from build123d import *

# Parameters (mm, degrees)
SKIZZE1_W                                 = 25
SKIZZE1_H                                 = 24
PCB_DEPTH                                 = 0.9
SKIZZE2_R                                 = 1.05
MOUNTING_HOLES_DEPTH                      = 20.165333287
SKIZZE3_W                                 = 20.8
SKIZZE3_H                                 = 5.5
CONNECTOR_CLOSED_DEPTH                    = 2.4
SKIZZE4_W                                 = 17.7
SKIZZE4_H                                 = 11.6
COMPONENTS_WORST_CASE_BOUNDARY_BOX_DEPTH  = 1.3
SKIZZE7_W                                 = 3
SKIZZE7_H                                 = 2
COMPONENTS_WORST_CASE_BOUNDARY_BOX2_DEPTH = 0.6
SKIZZE8_W                                 = 1.3
SKIZZE8_H                                 = 0.9
STATUS_LED_DEPTH                          = 0.01
ESBO_O1_R                                 = 3.5
RESSALTO_EXTRUS_O2_DEPTH                  = 3


with BuildPart() as part:
    # Skizze1 → PCB (new body)
    with BuildSketch(Plane(origin=(0, 0, 0), x_dir=(1, 0, 0), z_dir=(0, 1, 0))):
        with Locations((0, 2.5)):
            Rectangle(SKIZZE1_W, SKIZZE1_H)
    extrude(amount=-PCB_DEPTH)

    # Skizze2 → Mounting_Holes (cut, through all)
    with BuildSketch(Plane(origin=(0, 0, 0), x_dir=(1, 0, 0), z_dir=(0, 1, 0))):
        with Locations(Location((10.5, 12.5, 0), (0, 0, 270))):
            Circle(SKIZZE2_R)
        with Locations(Location((10.5, 0, 0), (0, 0, 270))):
            Circle(SKIZZE2_R)
        with Locations(Location((-10.5, 0, 0), (0, 0, 90))):
            Circle(SKIZZE2_R)
        with Locations(Location((-10.5, 12.5, 0), (0, 0, 90))):
            Circle(SKIZZE2_R)
    extrude(amount=-MOUNTING_HOLES_DEPTH, mode=Mode.SUBTRACT)

    # Skizze3 → Connector_closed (add)
    with BuildSketch(Plane.XZ.offset(0.9)):
        with Locations((0, 6.75)):
            Rectangle(SKIZZE3_W, SKIZZE3_H)
    extrude(amount=CONNECTOR_CLOSED_DEPTH)

    # Skizze4 → Components_worst-case_Boundary-Box (add)
    with BuildSketch(Plane.XZ.offset(0.9)):
        with Locations((-0.15, -6.7)):
            Rectangle(SKIZZE4_W, SKIZZE4_H)
    extrude(amount=COMPONENTS_WORST_CASE_BOUNDARY_BOX_DEPTH)

    # Skizze7 → Components_worst-case_Boundary-Box2 (add)
    with BuildSketch(Plane(origin=(0, 0, 0), x_dir=(1, 0, 0), z_dir=(0, 1, 0))):
        with Locations((7, 9.9)):
            Rectangle(SKIZZE7_W, SKIZZE7_H)
    extrude(amount=COMPONENTS_WORST_CASE_BOUNDARY_BOX2_DEPTH)

    # Skizze8 → Status_LED (cut)
    with BuildSketch(Plane(origin=(0, 0.6, 0), x_dir=(1, 0, 0), z_dir=(0, 1, 0))):
        with Locations((7.45, 9.45)):
            Rectangle(SKIZZE8_W, SKIZZE8_H)
    extrude(amount=-STATUS_LED_DEPTH, mode=Mode.SUBTRACT)

    # Esboço1 → Ressalto-extrusão2 (add)
    with BuildSketch(Plane(origin=(0, 0, 0), x_dir=(1, 0, 0), z_dir=(0, 1, 0))):
        with Locations(Location((0, 0, 0), (0, 0, 270))):
            Circle(ESBO_O1_R)
    extrude(amount=RESSALTO_EXTRUS_O2_DEPTH)


solid = part.part
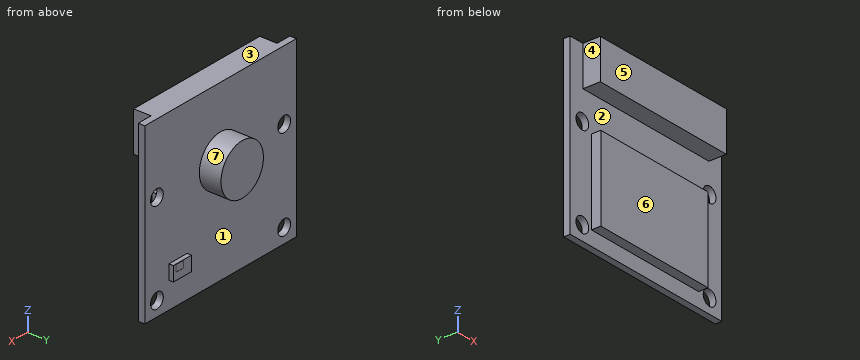
Could you check a few things on this model? Use its own coordinates, in mm. Face numbers are marked on the shaded views. A direction names the side the tool comes from. Coordinates: 2 decimals unless noted, no trailing zeros. Write each loop counter-clockwise with the first axis right and the second up, starting at its lowest first coordinate (ties: lowest second). Pieces come first, ordered by that corner, then holes. Notation, with made-up numbers: (61, 22) - (87, 22) arc R23 cw to (87, 44) - close; hole circle Ø3 at (-22.75, -3.5). An arc over 180 degrees is marked (long way). Write item = value, one per line.
1) Please list where these lines run through material, in increasing order: line 1 (X direction, y = -0.4, z = -12.5); line 2 (Z direction, x = -10.5, y = -0.55); line 3 (Z direction, x = -2.75, y = -1.25). Write a range as [from, to].
Result set:
line_1 = [-12.5, -11.55], [-9.45, 9.45], [11.55, 12.5]
line_2 = [-14.5, -13.55], [-11.45, -1.05], [1.05, 9.5]
line_3 = [-12.5, -0.9], [4, 9.5]
2) Suppose I cut it at C-C on z = 5.25. Please give me the cut outline in (x, y).
Result set:
outline = (-12.5, -0.9) - (-10.4, -0.9) - (-10.4, -3.3) - (10.4, -3.3) - (10.4, -0.9) - (12.5, -0.9) - (12.5, 0) - (-12.5, 0) - close
3) Suppose I cut it at D-D on x = 0. Please give me the cut outline in (y, z), plus the area to 3 significant figures.
Result set:
outline = (-3.3, 4) - (-0.9, 4) - (-0.9, -0.9) - (-2.2, -0.9) - (-2.2, -12.5) - (-0.9, -12.5) - (-0.9, -14.5) - (0, -14.5) - (0, -3.5) - (3, -3.5) - (3, 3.5) - (0, 3.5) - (0, 9.5) - (-3.3, 9.5) - close
area = 70.9 mm2
4) Suppose I cut it at A-A on z = 0. Please give me the cut outline in (x, y).
Result set:
outline = (-12.5, -0.9) - (-11.55, -0.9) - (-11.55, 0) - (-12.5, 0) - close; (-9.45, -0.9) - (9.45, -0.9) - (9.45, 0) - (3.5, 0) - (3.5, 3) - (-3.5, 3) - (-3.5, 0) - (-9.45, 0) - close; (11.55, -0.9) - (12.5, -0.9) - (12.5, 0) - (11.55, 0) - close
5) Will these pins go through, and if not, where does the flat tip stop? pin 1 Ø1 at (x, y) = (1.5, 1.5) entering from -Z; pin 2 Ø1.7 at (x, z) = (-10.5, -12.5) entering from +Y; pin 3 Ø1.5 at (y, z) = (-2.5, -10) entering from +X; pin 4 Ø0.5 at (y, z) = (0.5, -9.5) entering from +X.
Result set:
pin_1 = -3.35
pin_2 = through
pin_3 = 8.7
pin_4 = 8.5
6) We'd pull the mould along Z, two halves only. Please class the marked faces 1, 2 and 3: +Z half, -Z half, draft (parallel to the pull), parting line (faces both ways), or undercut.
Result set:
face_1 = draft
face_2 = undercut
face_3 = +Z half
7) Suppose I cut it at B-B on y = -1.25. Please give me the cut outline in (x, z).
Result set:
outline = (-10.4, 4) - (10.4, 4) - (10.4, 9.5) - (-10.4, 9.5) - close; (-9, -12.5) - (8.7, -12.5) - (8.7, -0.9) - (-9, -0.9) - close
8) For the marked faces 4, 5, 6 and 7, which set-ups out of +Z, -Z, +X, -X, +Y, -Y let a thin tool reach every point of the face, with its end or its side?
Result set:
face_4 = +Z, -Z, -X, -Y
face_5 = +Z, -Z, +X, -X, -Y
face_6 = -Z, +X, -X, -Y
face_7 = +Y
